```python
from build123d import *

# Parameters (mm, degrees)
SKETCH1_W               = 260.35
SKETCH1_H               = 107.95
BOSS_EXTRUDE1_DEPTH     = 6.35
SKETCH3_W               = 6.35
SKETCH3_H               = 6.35
CUT_EXTRUDE1_DEPTH      = 7.35
LPATTERN1_COUNT         = 8
LPATTERN1_PITCH         = 12.7
MIRROR1_COPY_1_SKETCH_W = 6.35
MIRROR1_COPY_1_SKETCH_H = 6.35
MIRROR1_COPY_1_DEPTH    = 7.35
MIRROR1_COPY_2_SKETCH_W = 6.35
MIRROR1_COPY_2_SKETCH_H = 6.35
MIRROR1_COPY_2_DEPTH    = 7.35
MIRROR1_COPY_3_SKETCH_W = 6.35
MIRROR1_COPY_3_SKETCH_H = 6.35
MIRROR1_COPY_3_DEPTH    = 7.35
MIRROR1_COPY_4_SKETCH_W = 6.35
MIRROR1_COPY_4_SKETCH_H = 6.35
MIRROR1_COPY_4_DEPTH    = 7.35
MIRROR1_COPY_5_SKETCH_W = 6.35
MIRROR1_COPY_5_SKETCH_H = 6.35
MIRROR1_COPY_5_DEPTH    = 7.35
MIRROR1_COPY_6_SKETCH_W = 6.35
MIRROR1_COPY_6_SKETCH_H = 6.35
MIRROR1_COPY_6_DEPTH    = 7.35
MIRROR1_COPY_7_SKETCH_W = 6.35
MIRROR1_COPY_7_SKETCH_H = 6.35
MIRROR1_COPY_7_DEPTH    = 7.35
SKETCH4_W               = 6.35
SKETCH4_H               = 6.35
CUT_EXTRUDE2_DEPTH      = 6.35
LPATTERN2_COUNT         = 21
LPATTERN2_PITCH         = 12.7


with BuildPart() as part:
    # Sketch1 → Boss-Extrude1 (new body)
    with BuildSketch(Plane.XY):
        Rectangle(SKETCH1_W, SKETCH1_H)
    extrude(amount=BOSS_EXTRUDE1_DEPTH)

    # Sketch3 → Cut-Extrude1 (cut, through all)
    with BuildSketch(Plane.XY.offset(6.35)):
        with Locations((127, -44.45)):
            Rectangle(SKETCH3_W, SKETCH3_H)
    cut_extrude1 = extrude(amount=-CUT_EXTRUDE1_DEPTH, mode=Mode.SUBTRACT)

    # LPattern1: Cut-Extrude1 ×8
    with Locations(*[(0, i * LPATTERN1_PITCH, 0) for i in range(1, LPATTERN1_COUNT)]):
        add(cut_extrude1, mode=Mode.SUBTRACT)

    # Mirror1: Cut-Extrude1 across plane
    add(cut_extrude1.mirror(Plane(origin=(0, 0, 0), x_dir=(0, 0, 1), z_dir=(1, 0, 0))), mode=Mode.SUBTRACT)

    # Mirror1 copy 1 sketch → Mirror1 copy 1 (cut, through all)
    with BuildSketch(Plane(origin=(0, 12.7, 6.35), x_dir=(-1, 0, 0), z_dir=(0, 0, 1))):
        with Locations((127, 44.45)):
            Rectangle(MIRROR1_COPY_1_SKETCH_W, MIRROR1_COPY_1_SKETCH_H)
    extrude(amount=-MIRROR1_COPY_1_DEPTH, mode=Mode.SUBTRACT)

    # Mirror1 copy 2 sketch → Mirror1 copy 2 (cut, through all)
    with BuildSketch(Plane(origin=(0, 25.4, 6.35), x_dir=(-1, 0, 0), z_dir=(0, 0, 1))):
        with Locations((127, 44.45)):
            Rectangle(MIRROR1_COPY_2_SKETCH_W, MIRROR1_COPY_2_SKETCH_H)
    extrude(amount=-MIRROR1_COPY_2_DEPTH, mode=Mode.SUBTRACT)

    # Mirror1 copy 3 sketch → Mirror1 copy 3 (cut, through all)
    with BuildSketch(Plane(origin=(0, 38.1, 6.35), x_dir=(-1, 0, 0), z_dir=(0, 0, 1))):
        with Locations((127, 44.45)):
            Rectangle(MIRROR1_COPY_3_SKETCH_W, MIRROR1_COPY_3_SKETCH_H)
    extrude(amount=-MIRROR1_COPY_3_DEPTH, mode=Mode.SUBTRACT)

    # Mirror1 copy 4 sketch → Mirror1 copy 4 (cut, through all)
    with BuildSketch(Plane(origin=(0, 50.8, 6.35), x_dir=(-1, 0, 0), z_dir=(0, 0, 1))):
        with Locations((127, 44.45)):
            Rectangle(MIRROR1_COPY_4_SKETCH_W, MIRROR1_COPY_4_SKETCH_H)
    extrude(amount=-MIRROR1_COPY_4_DEPTH, mode=Mode.SUBTRACT)

    # Mirror1 copy 5 sketch → Mirror1 copy 5 (cut, through all)
    with BuildSketch(Plane(origin=(0, 63.5, 6.35), x_dir=(-1, 0, 0), z_dir=(0, 0, 1))):
        with Locations((127, 44.45)):
            Rectangle(MIRROR1_COPY_5_SKETCH_W, MIRROR1_COPY_5_SKETCH_H)
    extrude(amount=-MIRROR1_COPY_5_DEPTH, mode=Mode.SUBTRACT)

    # Mirror1 copy 6 sketch → Mirror1 copy 6 (cut, through all)
    with BuildSketch(Plane(origin=(0, 76.2, 6.35), x_dir=(-1, 0, 0), z_dir=(0, 0, 1))):
        with Locations((127, 44.45)):
            Rectangle(MIRROR1_COPY_6_SKETCH_W, MIRROR1_COPY_6_SKETCH_H)
    extrude(amount=-MIRROR1_COPY_6_DEPTH, mode=Mode.SUBTRACT)

    # Mirror1 copy 7 sketch → Mirror1 copy 7 (cut, through all)
    with BuildSketch(Plane(origin=(0, 88.9, 6.35), x_dir=(-1, 0, 0), z_dir=(0, 0, 1))):
        with Locations((127, 44.45)):
            Rectangle(MIRROR1_COPY_7_SKETCH_W, MIRROR1_COPY_7_SKETCH_H)
    extrude(amount=-MIRROR1_COPY_7_DEPTH, mode=Mode.SUBTRACT)

    # Sketch4 → Cut-Extrude2 (cut)
    with BuildSketch(Plane.XY.offset(6.35)):
        with Locations((-127, 50.8)):
            Rectangle(SKETCH4_W, SKETCH4_H)
    cut_extrude2 = extrude(amount=-CUT_EXTRUDE2_DEPTH, mode=Mode.SUBTRACT)

    # LPattern2: Cut-Extrude2 ×21
    with Locations(*[(i * LPATTERN2_PITCH, 0, 0) for i in range(1, LPATTERN2_COUNT)]):
        add(cut_extrude2, mode=Mode.SUBTRACT)


solid = part.part
```
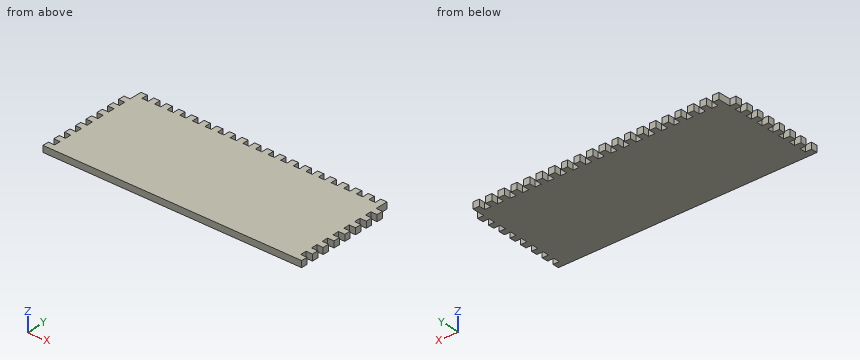
The model under review builds one solid part; all positions refer to its coordinate system, in mm. Round coordinates to 2 decimals unless told otherwise and drop trailing zeros. Loops run counter-clockwise (first coordinate to the right, second up) from the corner with the lowest first, then second, coordinate; pieces in that order, holes last.
1) Wall thickness on line 1 along X through (y, z) = (46, 3.5) (3 decimals); line 2 along Y through (x, z) = (-75.5, 4.75) (3 decimals): over which ranges is each line inside the solid? List them lowest first.
Values follow:
line 1: x = -123.825 to 123.825
line 2: y = -53.975 to 47.625
2) Consider section A-A on x = -77. State the section outline as (y, z) points (3 decimals).
Values follow:
outline: (-53.975, 0) - (47.625, 0) - (47.625, 6.35) - (-53.975, 6.35) - close
3) Clearance check with flat-ended pins moving along their axes: P1, Ø1.9, axis at y = 5, z = 3.5, coming from the +X side (3 decimals); P2, Ø3, axis at y = 49.5, z = 4.5, coming from the -X side (3 decimals); P3, Ø1, axis at x = -69.5, y = -12.5, coming from the -Z side; P4, Ø1.9, axis at x = 125.5, z = 3, coming from the +Y side (3 decimals). State where each tip first meets the part, or that it passes through.
Values follow:
P1: stops at x = 123.825
P2: stops at x = -123.825
P3: stops at z = 0
P4: stops at y = 41.275
